```python
from build123d import *

# Parameters (mm, degrees)
SKETCH1_R           = 39
SKETCH1_R_2         = 1.5
SKETCH1_R_3         = 7.5
BOSS_EXTRUDE1_DEPTH = 1
BOSS_EXTRUDE2_START = 9
SKETCH1_3_R         = 27.5
SKETCH1_3_R_2       = 1.5
SKETCH1_3_R_3       = 7.5
BOSS_EXTRUDE2_DEPTH = 9


with BuildPart() as part:
    # Sketch1 → Boss-Extrude1 (new body)
    with BuildSketch(Plane(origin=(0, 0, 0), x_dir=(1, 0, 0), z_dir=(0, 1, 0))):
        with Locations(Location((0, 0, 0), (0, 0, 270))):
            Circle(SKETCH1_R)
        with Locations(Location((22.5, 0, 0), (0, 0, 270))):
            Circle(SKETCH1_R_2, mode=Mode.SUBTRACT)
        with Locations(Location((15.909902577, -15.909902577, 0), (0, 0, 270))):
            Circle(SKETCH1_R_2, mode=Mode.SUBTRACT)
        with Locations(Location((0, -22.5, 0), (0, 0, 270))):
            Circle(SKETCH1_R_2, mode=Mode.SUBTRACT)
        with Locations(Location((-15.909902577, -15.909902577, 0), (0, 0, 270))):
            Circle(SKETCH1_R_2, mode=Mode.SUBTRACT)
        with Locations(Location((-22.5, 0, 0), (0, 0, 270))):
            Circle(SKETCH1_R_2, mode=Mode.SUBTRACT)
        with Locations(Location((-15.909902577, 15.909902577, 0), (0, 0, 270))):
            Circle(SKETCH1_R_2, mode=Mode.SUBTRACT)
        with Locations(Location((0, 22.5, 0), (0, 0, 270))):
            Circle(SKETCH1_R_2, mode=Mode.SUBTRACT)
        with Locations(Location((15.909902577, 15.909902577, 0), (0, 0, 270))):
            Circle(SKETCH1_R_2, mode=Mode.SUBTRACT)
        with Locations(Location((0, 0, 0), (0, 0, 270))):
            Circle(SKETCH1_R_3, mode=Mode.SUBTRACT)
    extrude(amount=-BOSS_EXTRUDE1_DEPTH)

    # Sketch1_3 → Boss-Extrude2 (add)
    with BuildSketch(Plane(origin=(0, 0, 0), x_dir=(1, 0, 0), z_dir=(0, 1, 0)).offset(BOSS_EXTRUDE2_START)):
        with Locations(Location((0, 0, 0), (0, 0, 270))):
            Circle(SKETCH1_3_R)
        with Locations(Location((-15.909902577, -15.909902577, 0), (0, 0, 270))):
            Circle(SKETCH1_3_R_2, mode=Mode.SUBTRACT)
        with Locations(Location((0, -22.5, 0), (0, 0, 270))):
            Circle(SKETCH1_3_R_2, mode=Mode.SUBTRACT)
        with Locations(Location((15.909902577, -15.909902577, 0), (0, 0, 270))):
            Circle(SKETCH1_3_R_2, mode=Mode.SUBTRACT)
        with Locations(Location((-22.5, 0, 0), (0, 0, 270))):
            Circle(SKETCH1_3_R_2, mode=Mode.SUBTRACT)
        with Locations(Location((-15.909902577, 15.909902577, 0), (0, 0, 270))):
            Circle(SKETCH1_3_R_2, mode=Mode.SUBTRACT)
        with Locations(Location((0, 22.5, 0), (0, 0, 270))):
            Circle(SKETCH1_3_R_2, mode=Mode.SUBTRACT)
        with Locations(Location((0, 0, 0), (0, 0, 270))):
            Circle(SKETCH1_3_R_3, mode=Mode.SUBTRACT)
        with Locations(Location((15.909902577, 15.909902577, 0), (0, 0, 270))):
            Circle(SKETCH1_3_R_2, mode=Mode.SUBTRACT)
        with Locations(Location((22.5, 0, 0), (0, 0, 270))):
            Circle(SKETCH1_3_R_2, mode=Mode.SUBTRACT)
    extrude(amount=-BOSS_EXTRUDE2_DEPTH)


solid = part.part
```
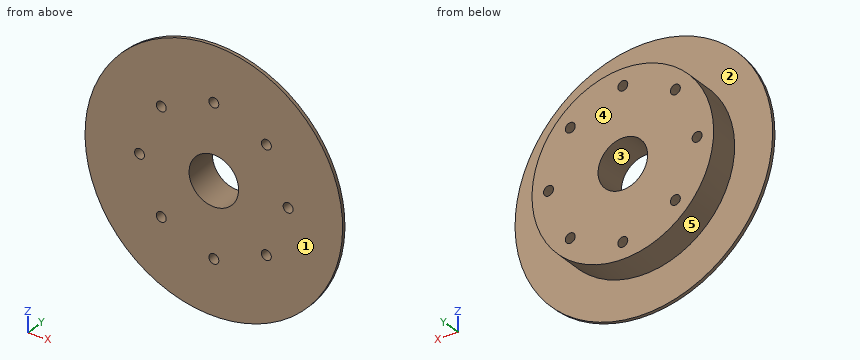
Part model, mm, in its own coordinate system. Face numbers are marked on the shaded views. A direction names the side the tool comes from. Round coordinates to 2 decimals unless told otherwise and drop trailing zeros. Loops run counter-clockwise (first coordinate to the right, second up) from the corner with the lowest first, then second, coordinate; pieces in that order, holes last.
1. Slice it at B-B (x = 0). Give the cut face in (y, z).
Solutions:
outline: (-1, -39) - (0, -39) - (0, -27.5) - (9, -27.5) - (9, -24) - (-1, -24) - close; (-1, -21) - (9, -21) - (9, -7.5) - (-1, -7.5) - close; (-1, 7.5) - (9, 7.5) - (9, 21) - (-1, 21) - close; (-1, 24) - (9, 24) - (9, 27.5) - (0, 27.5) - (0, 39) - (-1, 39) - close
2. Two-plate mould, pull along X, no slides. Class the marked faces 3, 4 and 5: pulls with the +X half, pulls with the -X half, needs draft (parallel to the pull), parting line crosses it, or undercut.
Solutions:
face 3: undercut
face 4: needs draft
face 5: parting line crosses it
3. Drill centre lines: line 1 along X through (y, z) = (4.75, 0); line 2 along X through (y, z) = (0.75, -17); line 3 along Z through (x, y) = (15, 7.5). Where is each one in solid material? Low to high.
Solutions:
line 1: x = -27.5 to -24, -21 to -7.5, 7.5 to 21, 24 to 27.5
line 2: x = -21.62 to -16.94, -14.88 to 14.88, 16.94 to 21.62
line 3: z = -23.05 to -17.1, -14.72 to 14.72, 17.1 to 23.05
4. Slice it at A-A (z = 0). Give the cut face in (x, y).
Solutions:
outline: (-39, -1) - (-24, -1) - (-24, 9) - (-27.5, 9) - (-27.5, 0) - (-39, 0) - close; (-21, -1) - (-7.5, -1) - (-7.5, 9) - (-21, 9) - close; (7.5, -1) - (21, -1) - (21, 9) - (7.5, 9) - close; (24, -1) - (39, -1) - (39, 0) - (27.5, 0) - (27.5, 9) - (24, 9) - close
5. Slice it at C-C (x = -22.5). Give the cut face in (y, z).
Solutions:
outline: (-1, -31.86) - (0, -31.86) - (0, -15.81) - (9, -15.81) - (9, -1.5) - (-1, -1.5) - close; (-1, 1.5) - (9, 1.5) - (9, 15.81) - (0, 15.81) - (0, 31.86) - (-1, 31.86) - close
6. Slice it at D-D (y = 2.5). Count the separate pieces of the cut face and the enclosed holes in it, and give its area (3 significant figures).
Solutions:
separate pieces: 1
enclosed holes: 9
area: 2,140 mm2
7. 3-axis set-ups, long thin cutter, end or side, ignore diameter. For the marked faces 1 and 2: which of +Z, -Z, +X, -X, +Y, -Y reach the whole face in a straight line?
Solutions:
face 1: +Z, -Z, +X, -X, -Y
face 2: +Y
8. Flat gauge pins, fed straight in: pin 1 (13.5 mm diameter, centred on x = 0, z = 0, fed in from +Y); pin 2 (6 mm diameter, centred on x = 26, y = 3.5, fed in from -Z); pin 3 (4 mm diameter, centred on x = -8, y = 6, fed in from +Z); pin 4 (5 mm diameter, centred on x = 15.5, y = 4.5, fed in from -Z). Where does each tip first touch, or does it go through?
Solutions:
pin 1: passes through
pin 2: stops at z = -15.07
pin 3: stops at z = 26.84
pin 4: stops at z = -24.23
